from build123d import *

# Parameters (mm, degrees)
SKETCH_W   = 80
SKETCH_H   = 40
SKETCH_R   = 12
SKETCH_R_2 = 1.5
PAD_DEPTH  = 3
FILLET_R   = 2


with BuildPart() as part:
    # Sketch → Pad (new body)
    with BuildSketch(Plane.XY):
        Rectangle(SKETCH_W, SKETCH_H)
        with Locations((-20, 0)):
            Circle(SKETCH_R, mode=Mode.SUBTRACT)
        with Locations((-35.5, 15.5)):
            Circle(SKETCH_R_2, mode=Mode.SUBTRACT)
        with Locations((-4.5, 15.5)):
            Circle(SKETCH_R_2, mode=Mode.SUBTRACT)
        with Locations((-35.5, -15.5)):
            Circle(SKETCH_R_2, mode=Mode.SUBTRACT)
        with Locations((-4.5, -15.5)):
            Circle(SKETCH_R_2, mode=Mode.SUBTRACT)
        with BuildLine():
            ThreePointArc((8, 1.5), (6.5, 0), (8, -1.5))
            Line((8, -1.5), (35, -1.5))
            ThreePointArc((35, -1.5), (36.5, 0), (35, 1.5))
            Line((8, 1.5), (35, 1.5))
        make_face(mode=Mode.SUBTRACT)
        with BuildLine():
            ThreePointArc((8, 8.5), (6.5, 7), (8, 5.5))
            Line((8, 5.5), (35, 5.5))
            ThreePointArc((35, 5.5), (36.5, 7), (35, 8.5))
            Line((8, 8.5), (35, 8.5))
        make_face(mode=Mode.SUBTRACT)
        with BuildLine():
            ThreePointArc((8, 15.5), (6.5, 14), (8, 12.5))
            Line((8, 12.5), (35, 12.5))
            ThreePointArc((35, 12.5), (36.5, 14), (35, 15.5))
            Line((8, 15.5), (35, 15.5))
        make_face(mode=Mode.SUBTRACT)
        with BuildLine():
            ThreePointArc((8, -5.5), (6.5, -7), (8, -8.5))
            Line((8, -8.5), (35, -8.5))
            ThreePointArc((35, -8.5), (36.5, -7), (35, -5.5))
            Line((8, -5.5), (35, -5.5))
        make_face(mode=Mode.SUBTRACT)
        with BuildLine():
            ThreePointArc((8, -12.5), (6.5, -14), (8, -15.5))
            Line((8, -15.5), (35, -15.5))
            ThreePointArc((35, -15.5), (36.5, -14), (35, -12.5))
            Line((8, -12.5), (35, -12.5))
        make_face(mode=Mode.SUBTRACT)
    extrude(amount=PAD_DEPTH)

    # Fillet
    fillet_edges = [part.edges().sort_by_distance(p)[0] for p in [
        (-40, 20, 1.5),
        (-40, -20, 1.5),
        (40, -20, 1.5),
        (40, 20, 1.5),
    ]]
    fillet(fillet_edges, radius=FILLET_R)


solid = part.part
CAD build for the part. Positions are in the model's coordinates, mm. A direction names the side the tool comes from. Coordinates: 2 decimals unless noted, no trailing zeros. Loops run counter-clockwise (first coordinate to the right, second up) from the corner with the lowest first, then second, coordinate; pieces in that order, holes last. Notation, with made-up numbers: (9, 59.25) - (30, 59.25) arc R11 ccw to (30, 73.25) - close; hole circle Ø3 at (31, 26.25). An arc over 180 degrees is marked (long way). Write item = value, one per line. Start each with the question number.
Q1. Cut at A-A, the plane x = -35.5. List the corners of the cut face in (y, z), then the cut area to 3 significant figures.
Q2. Cut at D-D, the plane z = 2.3. Give the number of separate pieces and of enclosed holes in the cut face, then the cut area to 3 significant figures.
Q3. Drill centre lines: L1, parallel to Y at x = -4.5, z = 1.15; L2, parallel to Y at x = 34, z = 0.8; L3, parallel to Y at x = -19.5, z = 2.85. Where is each one in solid material? Low to high.
Q4. Which spindle directions (+Z, -Z, +X, -X, +Y, -Y) get a long thin tool onto all of the face, cutting with end or side? Do faces 5 (the flat face through (21, 1.5, 1)), 6 (the flat face through (40, 0, 1)). Say none if no direction does.
Q5. Cut at B-B, the plane x = 25.5. List the corners of the cut face in (y, z), then the cut area to 3 significant figures.
Q6. Flat gauge pin, fed straight in: pin 1 Ø4 at (x, y) = (-35.5, 15.5) entering from +Z. Where does the tip first touch, or does it go through?
Q7. Cut at C-C, the plane y = 0. List the corners of the cut face in (x, z).
Q8. Pull direction Y, two halves, no side cores. Call faces 1 (the flat face through (21, 5.5, 1)), 2 (the flat face through (-1, 0, 3)), 3 (the flat face through (21, 8.5, 1)), 4 (the cylindrical face through (-39.43, -19.4, 1.52)): pulls with the +Y half, pulls with the -Y half, needs draft (parallel to the pull), parting line crosses it, or undercut.
Computed:
q1.outline = (-20, 0) - (-17, 0) - (-17, 3) - (-20, 3) - close; (-14, 0) - (14, 0) - (14, 3) - (-14, 3) - close; (17, 0) - (20, 0) - (20, 3) - (17, 3) - close
q1.area = 102 mm²
q2.separate_pieces = 1
q2.enclosed_holes = 10
q2.area = 2,280 mm²
q3.L1 = -20 to -17, -14 to 14, 17 to 20
q3.L2 = -20 to -15.5, -12.5 to -8.5, -5.5 to -1.5, 1.5 to 5.5, 8.5 to 12.5, 15.5 to 20
q3.L3 = -20 to -11.99, 11.99 to 20
q4.face_5 = +Z, -Z
q4.face_6 = +Z, -Z, +X, +Y, -Y
q5.outline = (-20, 0) - (-15.5, 0) - (-15.5, 3) - (-20, 3) - close; (-12.5, 0) - (-8.5, 0) - (-8.5, 3) - (-12.5, 3) - close; (-5.5, 0) - (-1.5, 0) - (-1.5, 3) - (-5.5, 3) - close; (1.5, 0) - (5.5, 0) - (5.5, 3) - (1.5, 3) - close; (8.5, 0) - (12.5, 0) - (12.5, 3) - (8.5, 3) - close; (15.5, 0) - (20, 0) - (20, 3) - (15.5, 3) - close
q5.area = 75.0 mm²
q6.pin_1 = 3
q7.outline = (-40, 0) - (-32, 0) - (-32, 3) - (-40, 3) - close; (-8, 0) - (6.5, 0) - (6.5, 3) - (-8, 3) - close; (36.5, 0) - (40, 0) - (40, 3) - (36.5, 3) - close
q8.face_1 = undercut
q8.face_2 = needs draft
q8.face_3 = undercut
q8.face_4 = pulls with the -Y half
